```python
from build123d import *

# Parameters (mm, degrees)
CUT_EXTRUDE1_DEPTH  = 21.72734614
CIRPATTERN1_COUNT   = 16
BOSS_EXTRUDE2_START = -4.412612
BOSS_EXTRUDE2_DEPTH = 80


with BuildPart() as part:
    # Sketch2 → Revolve1 (revolve)
    with BuildSketch(Plane(origin=(0, 0, 0), x_dir=(0, 0, -1), z_dir=(1, 0, 0))):
        Polygon((0, 0), (0, 4), (1, 9.299998774), (4.412612001, 8.617472191), (4.412612001, 0), align=None)
    revolve(axis=Axis((0, 0, -4.412612001), (0, 0, 1)))

    # Sketch6 → Cut-Extrude1 (cut, through all)
    with BuildSketch(Plane(origin=(0, 8.421354901, -5.393192445), x_dir=(-1, 0, 0), z_dir=(0, -0.19611729080207105, -0.9805804445574345))):
        with BuildLine():
            Line((-0.6, -2), (0.6, -2))
            ThreePointArc((0.6, -2), (1.069979771, -0.514520871), (1.75, 0.887299986))
            ThreePointArc((1.75, 0.887299986), (0, 1.049875288), (-1.75, 0.887299986))
            ThreePointArc((-1.75, 0.887299986), (-1.069979771, -0.514520871), (-0.6, -2))
        make_face()
    cut_extrude1 = extrude(amount=-CUT_EXTRUDE1_DEPTH, mode=Mode.SUBTRACT)

    # CirPattern1: Cut-Extrude1 ×16 about axis
    cirpattern1_axis = Axis((0, 0, 0), (0, 0, 1))
    for i in range(1, CIRPATTERN1_COUNT):
        add(cut_extrude1.rotate(cirpattern1_axis, i * 360 / CIRPATTERN1_COUNT), mode=Mode.SUBTRACT)

    # Sketch7 → Boss-Extrude2 (add)
    with BuildSketch(Plane(origin=(0, 0, -4.412612001), x_dir=(-1, 0, 0), z_dir=(0, 0, -1)).offset(BOSS_EXTRUDE2_START)):
        with BuildLine():
            Line((-1.92003444, 1.5), (1.92003444, 1.5))
            ThreePointArc((1.92003444, 1.5), (0, -2.4365), (-1.92003444, 1.5))
        make_face()
    extrude(amount=BOSS_EXTRUDE2_DEPTH)


solid = part.part
```
Can you work these out from the model? Positions are in its coordinate system, mm. A direction names the side the tool comes from. Coordinates: 2 decimals unless noted, no trailing zeros. Loops run counter-clockwise (first coordinate to the right, second up) from the corner with the lowest first, then second, coordinate; pieces in that order, holes last. Notation, with made-up numbers: (-16.75, -9) -> (36.25, -9) arc R14 cw to (36.25, 9) -> close; hole circle Ø9 at (15.5, 3.25). An arc over 180 degrees is marked (long way). Put each result on its own line as item: value. Start each with the question number.
Q1. I want a section at A-A (z = -20.5). Write out the boundary of the cut face in (x, y).
Q2. I'm going to push flat-ended pins straight in: P1, Ø1.2, axis at x = 0, z = -52, coming from the +Y side; P2, Ø6, axis at y = 1, z = -49.5, coming from the +X side; P3, Ø2, axis at y = -3, z = -68.5, coming from the +X side; P4, Ø6, axis at x = -6, z = -18, coming from the +Y side. Where does each tip first touch, or does it pass through?
Q3. Thinking about a two-plate mould opening in Y: for faces 1 (the face through (0.877, -7.893, -2.733)), 2 (the face through (-3.83, 6.957, -2.733)), 3 (the face through (6.419, -2.668, -2.547)), 4 (the face through (7.92, -0.886, -2.738)), which applies, pulls with the +Y half, pulls with the -Y half, needs draft (parallel to the pull), parting line crosses it, or undercut?
Q4. For faces 5 (the face through (0, 1.5, -42)), 6 (the face through (6.957, 3.83, -2.733)), 7 (the face through (-7.893, -0.877, -2.733)), 8 (the face through (-0.076, -2.435, -41.677)), which set-ups out of +Z, -Z, +X, -X, +Y, -Y let a thin tool reach every point of the face, with its end or its side?
Q5. If I drill on line 1 (Y direction, x = 1.5, z = -61); line 2 (Y direction, x = 0, z = -60); line 3 (Z direction, x = -4, y = -6.25), over which ranges is the centre line in solid material (lowest first)? Write a range as [from, to].
Taken from the geometry:
1. outline: (-1.92, 1.5) arc R2.44 ccw (long way) to (1.92, 1.5) -> close
2. P1: stops at y = 1.5
2. P2: stops at x = 2.44
2. P3: stops at x = 1.39
2. P4: passes through
3. face 1: pulls with the -Y half
3. face 2: pulls with the +Y half
3. face 3: undercut
3. face 4: undercut
4. face 5: -Z, +X, -X, +Y
4. face 6: -Z, +X
4. face 7: -Z, -X
4. face 8: -Z
5. line 1: y = [-1.92, 1.5]
5. line 2: y = [-2.44, 1.5]
5. line 3: z = [-4.41, -0.65]
